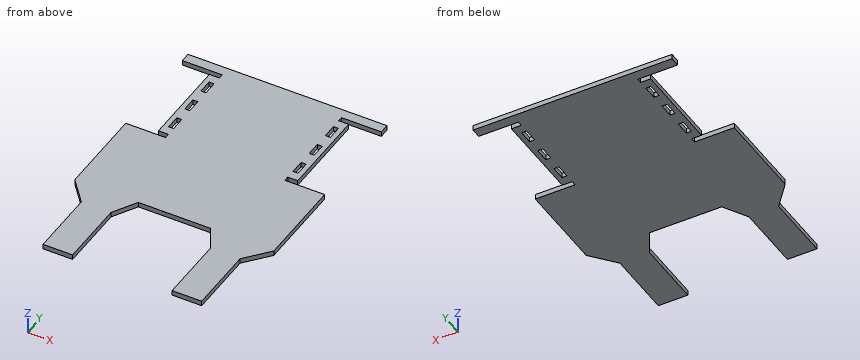
from build123d import *

# Parameters (mm, degrees)
F1_DEPTH = 3.175
F3_W     = 3.175
F3_H     = 9.0678
F4_DEPTH = 25.4
F6_DEPTH = 25.4


with BuildPart() as f1:
    # F0 (on Top) → F1 (new body)
    with BuildSketch(Plane.XY):
        Polygon((-50.681875, -44.462932), (-114.181875, -44.462932), (-114.181875, -171.462932), (-101.325941, -186.661884), (-101.325941, -229.702711), (-82.431875, -229.702711), (-82.431875, -186.661884), (-73.656756, -171.462932), (-50.681875, -171.462932), align=None)
        Polygon((12.818125, -44.462932), (-50.681875, -44.462932), (-50.681875, -171.462932), (-27.706994, -171.462932), (-18.931875, -186.661884), (-18.931875, -229.702711), (-0.03781, -229.702711), (-0.03781, -186.661884), (12.818125, -171.462932), align=None)
    extrude(amount=F1_DEPTH)

    # F3 (on face) → F4 (cut)
    with BuildSketch(Plane.XY.offset(3.175)):
        with Locations((-110.054375, -64.414632)):
            Rectangle(F3_W, F3_H)
        with Locations((-110.054375, -82.550232)):
            Rectangle(F3_W, F3_H)
        with Locations((-110.054375, -100.685832)):
            Rectangle(F3_W, F3_H)
        with Locations((-90.369375, -64.414632)):
            Rectangle(F3_W, F3_H)
        with Locations((-90.369375, -82.550232)):
            Rectangle(F3_W, F3_H)
        with Locations((-90.369375, -100.685832)):
            Rectangle(F3_W, F3_H)
        with Locations((-10.994375, -82.550232)):
            Rectangle(F3_W, F3_H)
        with Locations((-10.994375, -64.414632)):
            Rectangle(F3_W, F3_H)
        with Locations((8.690625, -100.685832)):
            Rectangle(F3_W, F3_H)
        with Locations((8.690625, -82.550232)):
            Rectangle(F3_W, F3_H)
        with Locations((-10.994375, -100.685832)):
            Rectangle(F3_W, F3_H)
        with Locations((8.690625, -64.414632)):
            Rectangle(F3_W, F3_H)
    extrude(amount=-F4_DEPTH, mode=Mode.SUBTRACT)

    # F5 (on face) → F6 (cut)
    with BuildSketch(Plane.XY.offset(3.175)):
        Polygon((-95.131875, -50.812932), (-114.181875, -50.812932), (-114.181875, -114.312932), (-95.131875, -114.312932), (-88.781875, -114.312932), (-88.781875, -111.137932), (-95.131875, -111.137932), (-95.131875, -53.987932), (-88.781875, -53.987932), (-88.781875, -50.812932), align=None)
        Polygon((-12.581875, -111.137932), (-12.581875, -114.312932), (-6.231875, -114.312932), (12.818125, -114.312932), (12.818125, -50.812932), (-6.231875, -50.812932), (-12.581875, -50.812932), (-12.581875, -53.987932), (-6.231875, -53.987932), (-6.231875, -111.137932), align=None)
    extrude(amount=-F6_DEPTH, mode=Mode.SUBTRACT)


solid = f1.part
The model under review builds one solid part; all positions refer to its coordinate system, in mm. Round coordinates to 2 decimals unless told otherwise and drop trailing zeros. Loops run counter-clockwise (first coordinate to the right, second up) from the corner with the lowest first, then second, coordinate; pieces in that order, holes last. Notation, with made-up numbers: (64, 31.25) -> (111, 31.25) arc R16 cw to (111, 51.25) -> close; hole circle Ø10 at (24.25, 12). An arc over 180 degrees is marked (long way). Write item = value, one per line. Start each with the question number.
Item 1: Take a section at A-A on y = -82. Give the boundary of the cut face in (x, z) (3 decimals), plus the area to 3 significant figures.
Item 2: To check wall thickness, follow L1, parallel to Y at x = -9.5, z = 2.3; L2, parallel to X at y = -80.5, z = 2.65; L3, parallel to X at y = -221, z = 0.25. State the ranges of each line that lie inside material, in increasing order.
Item 3: Take a section at C-C on x = 2.5. Give the boundary of the cut face in (y, z) (3 decimals), plus the area to 3 significant figures.
Item 4: Take a section at B-B on y = -198. Give the boundary of the cut face in (x, z) (3 decimals).
Item 5: Take a section at D-D on z = 0.75. Count the separate pieces of the cut face and the enclosed holes in it, plus the area to 3 significant figures.
Item 6: Insertion check: pin 1 (1.6 mm diameter, centred on x = 5, z = 1.5, fed in from -Y); pin 2 (1.6 mm diameter, centred on y = -102, z = 2, fed in from +X); pin 3 (5 mm diameter, centred on x = -1.5, y = -149.5, fed in from -Z); pin 4 (1 mm diameter, centred on y = -52, z = 1.5, fed in from -X). Each pin has a flat end and moves straight along its axis. Give the tip position at first contact, or say it passes through.
Result:
q1.outline = (-95.132, 0) -> (-91.957, 0) -> (-91.957, 3.175) -> (-95.132, 3.175) -> close; (-88.782, 0) -> (-12.582, 0) -> (-12.582, 3.175) -> (-88.782, 3.175) -> close; (-9.407, 0) -> (-6.232, 0) -> (-6.232, 3.175) -> (-9.407, 3.175) -> close
q1.area = 262 mm²
q2.L1 = -229.7 to -114.31, -111.14 to -105.22, -96.15 to -87.08, -78.02 to -68.95, -59.88 to -53.99, -50.81 to -44.46
q2.L2 = -95.13 to -91.96, -88.78 to -12.58, -9.41 to -6.23
q2.L3 = -101.33 to -82.43, -18.93 to -0.04
q3.outline = (-183.662, 0) -> (-114.313, 0) -> (-114.313, 3.175) -> (-183.662, 3.175) -> close; (-50.813, 0) -> (-44.463, 0) -> (-44.463, 3.175) -> (-50.813, 3.175) -> close
q3.area = 240 mm²
q4.outline = (-101.326, 0) -> (-82.432, 0) -> (-82.432, 3.175) -> (-101.326, 3.175) -> close; (-18.932, 0) -> (-0.038, 0) -> (-0.038, 3.175) -> (-18.932, 3.175) -> close
q5.separate_pieces = 1
q5.enclosed_holes = 6
q5.area = 16,000 mm²
q6.pin_1 = -181.65
q6.pin_2 = -6.23
q6.pin_3 = 0
q6.pin_4 = -88.78
